Here's how the part is built. I have some questions about the finished solid (model axes, mm). Round coordinates to 2 decimals unless told otherwise and drop trailing zeros. Write each loop counter-clockwise with the first axis right and the second up, starting at its lowest first coordinate (ties: lowest second). Pieces come first, ordered by that corner, then holes. Notation, with made-up numbers: M 61.5,-4 L 107.5,-4 A22 cw 107.5,12 Z; hole C 81.5,21 d5. An arc over 180 degrees is marked long. Write item = value, one per line. Start each with the question number.
(1) I need wall thicknesses on line 1 along Y through (x, z) = (82, 2.25); line 2 along Y through (x, z) = (-70, 1.25); line 3 along X through (y, z) = (16.5, 2). Which ranges of each line are inside material? Lowest first, please.
(2) Will these pins go through, and if not, where does the flat tip stop? pin 1 Ø1.5 at (x, z) = (123.5, 2.5) entering from +Y; pin 2 Ø4 at (y, z) = (-20.5, 7) entering from +X; pin 3 Ø11.5 at (x, y) = (-74.51, 79.9) entering from +Z; pin 4 Ø9 at (x, y) = (-103.1, 36.12) entering from +Z.
(3) I want a section at A-A (z = 5.75). List the corners of the cut face in (x, y) for me.
```python
from build123d import *

# Parameters (mm, degrees)
SKETCH1_R           = 155
SKETCH1_R_2         = 30
EXTRUDE_THIN1_DEPTH = 3
SKETCH3_R           = 40
SKETCH3_R_2         = 30
EXTRUDE_THIN2_DEPTH = 5
SKETCH7_R           = 5
CUT_EXTRUDE3_DEPTH  = 220.260119493
SKETCH9_R           = 2.5
CUT_EXTRUDE4_DEPTH  = 220.349036925


with BuildPart() as part:
    # Sketch1 → Extrude-Thin1 (new body)
    with BuildSketch(Plane.XY):
        Circle(SKETCH1_R)
        Circle(SKETCH1_R_2, mode=Mode.SUBTRACT)
    extrude(amount=EXTRUDE_THIN1_DEPTH)

    # Sketch3 → Extrude-Thin2 (add)
    with BuildSketch(Plane.XY.offset(3)):
        Circle(SKETCH3_R)
        Circle(SKETCH3_R_2, mode=Mode.SUBTRACT)
    extrude(amount=EXTRUDE_THIN2_DEPTH)

    # Sketch7 → Cut-Extrude3 (cut, through all)
    with BuildSketch(Plane.XY.offset(3)):
        with Locations((-50.351181472, 45.541803602)):
            Circle(SKETCH7_R)
        with Locations((-58.402643714, 56.994923516)):
            Circle(SKETCH7_R)
        with Locations((-66.454105956, 68.44804343)):
            Circle(SKETCH7_R)
        with Locations((-74.505568198, 79.901163345)):
            Circle(SKETCH7_R)
        with Locations((-82.55703044, 91.354283259)):
            Circle(SKETCH7_R)
        with Locations((-23.419425603, 63.724625189)):
            Circle(SKETCH7_R)
        with Locations((-25.226111144, 77.607560302)):
            Circle(SKETCH7_R)
        with Locations((-27.032796685, 91.490495415)):
            Circle(SKETCH7_R)
        with Locations((-28.839482226, 105.373430528)):
            Circle(SKETCH7_R)
        with Locations((-30.646167767, 119.256365641)):
            Circle(SKETCH7_R)
        with Locations((8.877438438, 67.308903109)):
            Circle(SKETCH7_R)
        with Locations((13.729419482, 80.441240295)):
            Circle(SKETCH7_R)
        with Locations((18.581400526, 93.57357748)):
            Circle(SKETCH7_R)
        with Locations((23.43338157, 106.705914665)):
            Circle(SKETCH7_R)
        with Locations((28.285362614, 119.83825185)):
            Circle(SKETCH7_R)
        with Locations((39.140588317, 55.473522488)):
            Circle(SKETCH7_R)
        with Locations((49.539705562, 64.846801558)):
            Circle(SKETCH7_R)
        with Locations((59.938822807, 74.220080628)):
            Circle(SKETCH7_R)
        with Locations((70.337940052, 83.593359698)):
            Circle(SKETCH7_R)
        with Locations((80.737057297, 92.966638768)):
            Circle(SKETCH7_R)
        with Locations((60.437101108, 30.929826393)):
            Circle(SKETCH7_R)
        with Locations((74.001042116, 34.396742073)):
            Circle(SKETCH7_R)
        with Locations((87.564983124, 37.863657753)):
            Circle(SKETCH7_R)
        with Locations((101.128924132, 41.330573433)):
            Circle(SKETCH7_R)
        with Locations((114.69286514, 44.797489113)):
            Circle(SKETCH7_R)
        with Locations((67.888202381, -0.699520184)):
            Circle(SKETCH7_R)
        with Locations((81.50963173, -3.933196495)):
            Circle(SKETCH7_R)
        with Locations((95.131061079, -7.166872806)):
            Circle(SKETCH7_R)
        with Locations((108.752490428, -10.400549118)):
            Circle(SKETCH7_R)
        with Locations((122.373919778, -13.634225429)):
            Circle(SKETCH7_R)
        with Locations((59.78693463, -32.168615117)):
            Circle(SKETCH7_R)
        with Locations((70.345347013, -41.362087146)):
            Circle(SKETCH7_R)
        with Locations((80.903759395, -50.555559176)):
            Circle(SKETCH7_R)
        with Locations((91.462171778, -59.749031206)):
            Circle(SKETCH7_R)
        with Locations((102.02058416, -68.942503236)):
            Circle(SKETCH7_R)
        with Locations((37.989200666, -56.268268)):
            Circle(SKETCH7_R)
        with Locations((43.065791048, -69.3154221)):
            Circle(SKETCH7_R)
        with Locations((48.14238143, -82.362576199)):
            Circle(SKETCH7_R)
        with Locations((53.218971811, -95.409730299)):
            Circle(SKETCH7_R)
        with Locations((58.295562193, -108.456884398)):
            Circle(SKETCH7_R)
        with Locations((7.488598649, -67.477538791)):
            Circle(SKETCH7_R)
        with Locations((5.920381353, -81.389429191)):
            Circle(SKETCH7_R)
        with Locations((4.352164057, -95.301319592)):
            Circle(SKETCH7_R)
        with Locations((2.783946761, -109.213209992)):
            Circle(SKETCH7_R)
        with Locations((1.215729465, -123.125100392)):
            Circle(SKETCH7_R)
        with Locations((-24.727551071, -63.228518637)):
            Circle(SKETCH7_R)
        with Locations((-32.581316361, -74.818098904)):
            Circle(SKETCH7_R)
        with Locations((-40.435081651, -86.407679171)):
            Circle(SKETCH7_R)
        with Locations((-48.288846942, -97.997259438)):
            Circle(SKETCH7_R)
        with Locations((-56.142612232, -109.586839705)):
            Circle(SKETCH7_R)
        with Locations((-51.27891684, -44.49460685)):
            Circle(SKETCH7_R)
        with Locations((-63.619027145, -51.106843814)):
            Circle(SKETCH7_R)
        with Locations((-75.959137449, -57.719080778)):
            Circle(SKETCH7_R)
        with Locations((-88.299247754, -64.331317742)):
            Circle(SKETCH7_R)
        with Locations((-100.639358059, -70.943554706)):
            Circle(SKETCH7_R)
        with Locations((-66.082900739, -15.567516851)):
            Circle(SKETCH7_R)
        with Locations((-80.082385502, -15.68762671)):
            Circle(SKETCH7_R)
        with Locations((-94.081870264, -15.807736569)):
            Circle(SKETCH7_R)
        with Locations((-108.081355027, -15.927846427)):
            Circle(SKETCH7_R)
        with Locations((-122.08083979, -16.047956286)):
            Circle(SKETCH7_R)
        with Locations((-78.199834438, 23.325436617)):
            Circle(SKETCH7_R)
        with Locations((-90.651580411, 29.724969584)):
            Circle(SKETCH7_R)
        with Locations((-103.103326385, 36.124502552)):
            Circle(SKETCH7_R)
        with Locations((-115.555072359, 42.52403552)):
            Circle(SKETCH7_R)
    extrude(amount=-CUT_EXTRUDE3_DEPTH, mode=Mode.SUBTRACT)

    # Sketch9 → Cut-Extrude4 (cut, through all)
    with BuildSketch(Plane.XY.offset(8)):
        with Locations((0, 35)):
            Circle(SKETCH9_R)
        with Locations((30.310889132, 17.5)):
            Circle(SKETCH9_R)
        with Locations((30.310889132, -17.5)):
            Circle(SKETCH9_R)
        with Locations((0, -35)):
            Circle(SKETCH9_R)
        with Locations((-30.310889132, -17.5)):
            Circle(SKETCH9_R)
        with Locations((-30.310889132, 17.5)):
            Circle(SKETCH9_R)
    extrude(amount=-CUT_EXTRUDE4_DEPTH, mode=Mode.SUBTRACT)


solid = part.part
```
Returned:
q1.line_1 = -131.53 to -55.43, -45.68 to -8.91, 1.04 to 88.13, 97.8 to 131.53
q1.line_2 = -138.29 to -18.67, -12.46 to 64.92, 71.97 to 77.73, 82.07 to 138.29
q1.line_3 = -154.12 to -32.6, -28.02 to -25.05, 25.05 to 28.02, 32.6 to 154.12
q2.pin_1 = 94.64
q2.pin_2 = 35.46
q2.pin_3 = 3
q2.pin_4 = through
q3.outline = C 0,0 d80; hole C -30.31,-17.5 d5; hole C -30.31,17.5 d5; hole C 0,0 d60; hole C 0,-35 d5; hole C 0,35 d5; hole C 30.31,-17.5 d5; hole C 30.31,17.5 d5
